from build123d import *

# Parameters (mm, degrees)
SKETCH_1_W          = 103.2
SKETCH_1_H          = 90.7
SKETCH_1_W_2        = 56.5
SKETCH_1_H_2        = 71.5
EXTRUDE_1_DEPTH     = 43
EXTRUDE_3_DEPTH     = 5
SKETCH_4_R          = 3.682623049
SKETCH_4_W          = 20.371137154
SKETCH_4_H          = 17.709581546
SKETCH_4_W_2        = 16.685906313
SKETCH_4_H_2        = 21.804282482
SKETCH_4_W_3        = 16.276436219
SKETCH_4_H_3        = 17.19774393
SKETCH_4_W_4        = 16.993008883
CUT_EXTRUDE_2_DEPTH = 4.377522815
SKETCH_5_W          = 4.606538552
SKETCH_5_H          = 28.355803979
CUT_EXTRUDE_3_DEPTH = 4.922477185
SKETCH_8_W          = 15
SKETCH_8_H          = 15
CUT_EXTRUDE_5_DEPTH = 15


with BuildPart() as part:
    # 草图1 → 凸台-拉伸1 (new body)
    with BuildSketch(Plane.XY):
        with BuildLine():
            Line((0, 10), (0, 39.186569494))
            ThreePointArc((0, 39.186569494), (1.375838219, 44.248568464), (5.124766715, 47.917669105))
            Line((5.124766715, 47.917669105), (10, 50.639880584))
            Line((10, 50.639880584), (10, 90))
            ThreePointArc((10, 90), (12.928932188, 97.071067812), (20, 100))
            Line((20, 100), (190, 100))
            ThreePointArc((190, 100), (197.071067812, 97.071067812), (200, 90))
            Line((200, 90), (200, 51.963395008))
            Line((200, 51.963395008), (205.683304945, 48.037782396))
            ThreePointArc((205.683304945, 48.037782396), (208.855310538, 44.455580593), (210, 39.809778695))
            Line((210, 39.809778695), (210, 10))
            ThreePointArc((210, 10), (207.071067812, 2.928932188), (200, 0))
            Line((200, 0), (10, 0))
            ThreePointArc((10, 0), (2.928932188, 2.928932188), (0, 10))
        make_face()
        with Locations((72.614593403, 50.272477185)):
            Rectangle(SKETCH_1_W, SKETCH_1_H, mode=Mode.SUBTRACT)
        with Locations((161.079111209, 50.675353005)):
            Rectangle(SKETCH_1_W_2, SKETCH_1_H_2, mode=Mode.SUBTRACT)
    extrude(amount=EXTRUDE_1_DEPTH)

    # 草图3 → 凸台-拉伸3 (add)
    with BuildSketch(Plane.XY):
        with BuildLine():
            Line((0, 10), (0, 39.186569494))
            ThreePointArc((0, 39.186569494), (1.375838219, 44.248568464), (5.124766715, 47.917669105))
            Line((5.124766715, 47.917669105), (10, 50.639880584))
            Line((10, 50.639880584), (10, 90))
            ThreePointArc((10, 90), (12.928932188, 97.071067812), (20, 100))
            Line((20, 100), (180, 100))
            ThreePointArc((180, 100), (187.071067812, 97.071067812), (190, 90))
            Line((190, 90), (190, 51.963395008))
            Line((190, 51.963395008), (195.683304945, 48.037782396))
            ThreePointArc((195.683304945, 48.037782396), (198.855310538, 44.455580593), (200, 39.809778695))
            Line((200, 39.809778695), (200, 10))
            ThreePointArc((200, 10), (197.071067812, 2.928932188), (190, 0))
            Line((190, 0), (10, 0))
            ThreePointArc((10, 0), (2.928932188, 2.928932188), (0, 10))
        make_face()
    extrude(amount=EXTRUDE_3_DEPTH)

    # 草图4 → 切除-拉伸2 (cut)
    with BuildSketch(Plane(origin=(0, 100, 0), x_dir=(1, 0, 0), z_dir=(0, 1, 0))):
        with Locations(Location((113.563696849, -10.32262821, 0), (0, 0, 180))):
            Circle(SKETCH_4_R)
        with Locations((141.053854619, -16.426982565)):
            Rectangle(SKETCH_4_W, SKETCH_4_H)
        with Locations((39.603161201, -18.474333033)):
            Rectangle(SKETCH_4_W_2, SKETCH_4_H_2)
        with Locations((67.958965179, -14.942653476)):
            Rectangle(SKETCH_4_W_3, SKETCH_4_H_3)
        with Locations((95.751747779, -14.942653476)):
            Rectangle(SKETCH_4_W_4, SKETCH_4_H_3)
    extrude(amount=-CUT_EXTRUDE_2_DEPTH, mode=Mode.SUBTRACT)

    # 草图5 → 切除-拉伸3 (cut)
    with BuildSketch(Plane.XZ):
        with Locations((34.452767739, 20.30710257)):
            Rectangle(SKETCH_5_W, SKETCH_5_H)
        with Locations((24.452767739, 20.30710257)):
            Rectangle(SKETCH_5_W, SKETCH_5_H)
        with Locations((44.452767739, 20.30710257)):
            Rectangle(SKETCH_5_W, SKETCH_5_H)
        with Locations((54.452767739, 20.30710257)):
            Rectangle(SKETCH_5_W, SKETCH_5_H)
        with Locations((64.452767739, 20.30710257)):
            Rectangle(SKETCH_5_W, SKETCH_5_H)
        with Locations((74.452767739, 20.30710257)):
            Rectangle(SKETCH_5_W, SKETCH_5_H)
        with Locations((84.452767739, 20.30710257)):
            Rectangle(SKETCH_5_W, SKETCH_5_H)
        with Locations((94.452767739, 20.30710257)):
            Rectangle(SKETCH_5_W, SKETCH_5_H)
    extrude(amount=-CUT_EXTRUDE_3_DEPTH, mode=Mode.SUBTRACT)

    # 草图8 → 切除-拉伸5 (cut)
    with BuildSketch(Plane.ZY):
        with Locations((35.5, 17.5)):
            Rectangle(SKETCH_8_W, SKETCH_8_H)
    cut_extrude_5 = extrude(amount=-CUT_EXTRUDE_5_DEPTH, mode=Mode.SUBTRACT)

    # 镜向1: 切除-拉伸5 across plane
    add(cut_extrude_5.mirror(Plane.ZY.offset(-105)), mode=Mode.SUBTRACT)


solid = part.part
The listing builds one solid part. Answer for the finished solid, in the listing's coordinates (mm). A direction names the side the tool comes from. Coordinates: 2 decimals unless noted, no trailing zeros. Write each loop counter-clockwise with the first axis right and the second up, starting at its lowest first coordinate (ties: lowest second). Pieces come first, ordered by that corner, then holes. Notation, with made-up numbers: M 35.25,-8.75 L 61.25,-8.75 A28 cw 61.25,22.25 Z; hole C 27,65 d7. An arc over 180 degrees is marked long. Use one line per item in the form item = value.
Item 1: Given P1, Ø19.5, axis at y = 74, z = 15.5, coming from the -X side; P2, Ø2, axis at y = 98.5, z = 14, coming from the -X side; P3, Ø4, axis at x = 111.5, y = 48.5, coming from the -Z side; P4, Ø2.5, axis at y = 3, z = 24, coming from the +X side, each flat-ended and moving along its own axis, determine where each tip first touches the part or whether it passes through.
Model answer:
P1 = 10
P2 = 13.39
P3 = 0
P4 = 208.18
Item 2: Find section B-B, the plane x = 114.5. Give the vertices of the cut face in (y, z).
Model answer:
outline = M 0,0 L 100,0 L 100,6.76 L 95.62,6.76 L 95.62,5 L 4.92,5 L 4.92,43 L 0,43 Z; M 95.62,13.88 L 100,13.88 L 100,43 L 95.62,43 Z
Item 3: Find section C-C, the plane y = 23. Give the vertices of the cut face in (x, z).
Model answer:
outline = M 0,0 L 210,0 L 210,28 L 195,28 L 195,43 L 189.33,43 L 189.33,5 L 132.83,5 L 132.83,43 L 124.21,43 L 124.21,5 L 21.01,5 L 21.01,43 L 15,43 L 15,28 L 0,28 Z
Item 4: The mould has two halves that part along Y. Classify faces 3 (the face through (36.756, 2, 20)), 4 (the face through (207.15, 3.01, 21.2)), 5 (the face through (15, 18, 35)), 6 (the face through (203, 25, 35)): released by +Y, released by -Y, zero draft, split by the parting line, or undercut.
Model answer:
face_3 = zero draft
face_4 = released by -Y
face_5 = undercut
face_6 = undercut
Item 5: For faces 1 (the face through (59.821, 98, 15)), 2 (the face through (64, 2, 34.485)), determine the directions among +Z, -Z, +X, -X, +Y, -Y from which every point of the face is accessible in a straight line to the end or side of a thin tool.
Model answer:
face_1 = +Y
face_2 = -Y
Item 6: Find section A-A, the plane z = 39.5. Give the vertices of the cut face in (x, y), plus the area to 3 significant figures.
Model answer:
outline = M 0,10 A10 ccw 10,0 L 200,0 A10 ccw 210,10 L 195,10 L 195,25 L 210,25 L 210,39.81 A10 ccw 205.68,48.04 L 200,51.96 L 200,90 A10 ccw 190,100 L 20,100 A10 ccw 10,90 L 10,50.64 L 5.12,47.92 A10 ccw 0,39.19 L 0,25 L 15,25 L 15,10 Z; hole M 21.01,4.92 L 124.21,4.92 L 124.21,95.62 L 21.01,95.62 Z; hole M 132.83,14.93 L 189.33,14.93 L 189.33,86.43 L 132.83,86.43 Z
area = 6,020 mm2
Item 7: Find the intervals of material crossed by probe 1 along X at (y, z) = (53.5, 38); probe 2 along X at (y, z) = (39, 27.5); probe 3 along X at (y, z) = (88.5, 19.5), in increasing order.
Model answer:
probe_1 = 10 to 21.01, 124.21 to 132.83, 189.33 to 200
probe_2 = 0 to 21.01, 124.21 to 132.83, 189.33 to 210
probe_3 = 10 to 21.01, 124.21 to 200
Item 8: Find section D-D, the plane x = 159.5. Give the vertices of the cut face in (y, z), plus the area to 3 significant figures.
Model answer:
outline = M 0,0 L 100,0 L 100,43 L 86.43,43 L 86.43,5 L 14.93,5 L 14.93,43 L 0,43 Z
area = 1,580 mm2
